Build history of the part. All positions in model axes, mm. Face numbers are marked on the shaded views. A direction names the side the tool comes from. Round coordinates to 2 decimals unless told otherwise and drop trailing zeros. Order: outer loops, then holes, each group sorted by start corner. A loop starts at its lowest first (then second) coordinate and runs counter-clockwise, first axis right, second up. Notation, with made-up numbers: (1, -35.75) - (19, -35.75) arc R20 ccw to (19, -12.75) - close; hole circle Ø8 at (-20.5, 85.25). An arc over 180 degrees is marked (long way). One line per question, with ' | ' between items. Start each with the question number.
from build123d import *

# Parameters (mm, degrees)
SKETCH11_W          = 38.1
SKETCH11_H          = 38.1
SKETCH12_W          = 38.1
SKETCH12_H          = 38.1
BOSS_EXTRUDE5_DEPTH = 12.7
BOSS_EXTRUDE5_TAPER = 20
BOSS_EXTRUDE6_DEPTH = 38.1
SKETCH15_R          = 12.065
CUT_EXTRUDE3_DEPTH  = 25.4
SKETCH16_W          = 23.310601064
SKETCH16_H          = 76.2
CUT_EXTRUDE4_DEPTH  = 59.830675793
SKETCH17_R          = 7.62
BOSS_EXTRUDE7_DEPTH = 6.35
SKETCH18_R          = 5.08
BOSS_EXTRUDE8_DEPTH = 3.81
SKETCH19_R          = 3.1115
BOSS_EXTRUDE9_DEPTH = 7.62
FILLET2_R           = 5.08
SKETCH21_R          = 1.35
CUT_EXTRUDE5_DEPTH  = 63.348983198


with BuildPart() as part:
    # Sweep1: sweep along a path in Sketch10
    with BuildLine(Plane(origin=(0, 0, 0), x_dir=(0, 0, -1), z_dir=(1, 0, 0))) as sweep1_path:
        Line((0, 96.393), (0, -5.207))
        Line((0, -5.207), (-25.324322261, -30.531322261))
    # Sketch11 → Sweep1 (sweep)
    with BuildSketch(Plane(origin=(0, 96.393, 0), x_dir=(1, 0, 0), z_dir=(0, 1, 0))):
        Rectangle(SKETCH11_W, SKETCH11_H)
    sweep(path=sweep1_path.line, transition=Transition.RIGHT)

    # Sketch12 → Boss-Extrude5 (add)
    with BuildSketch(Plane(origin=(0, -27.927822261, 27.927822261), x_dir=(1, 0, 0), z_dir=(0, -0.7071067811865461, 0.7071067811865489))):
        with Locations((0, -3.68190501)):
            Rectangle(SKETCH12_W, SKETCH12_H)
    extrude(amount=BOSS_EXTRUDE5_DEPTH, taper=BOSS_EXTRUDE5_TAPER)

    # Sketch13 → Boss-Extrude6 (add)
    with BuildSketch(Plane(origin=(0, 0, -19.05), x_dir=(-1, 0, 0), z_dir=(0, 0, -1))):
        with BuildLine():
            Line((-19.05, 96.393), (19.05, 96.393))
            ThreePointArc((19.05, 96.393), (0, 115.443), (-19.05, 96.393))
        make_face()
    extrude(amount=-BOSS_EXTRUDE6_DEPTH)

    # Sketch15 → Cut-Extrude3 (cut)
    with BuildSketch(Plane(origin=(0, -36.908078382, 36.908078382), x_dir=(1, 0, 0), z_dir=(0, -0.7071067811865461, 0.7071067811865489))):
        with Locations(Location((0, -3.68190501, 0), (0, 0, 270))):
            Circle(SKETCH15_R)
    extrude(amount=-CUT_EXTRUDE3_DEPTH, mode=Mode.SUBTRACT)

    # Sketch16 → Cut-Extrude4 (cut)
    with BuildSketch(Plane(origin=(19.05, 0, 0), x_dir=(0, 0, -1), z_dir=(1, 0, 0))):
        with Locations((0, 45.72)):
            Rectangle(SKETCH16_W, SKETCH16_H)
    extrude(amount=-CUT_EXTRUDE4_DEPTH, mode=Mode.SUBTRACT)

    # Sketch17 → Boss-Extrude7 (add)
    with BuildSketch(Plane.XY.offset(19.05)):
        with Locations(Location((0, 96.393, 0), (0, 0, 90))):
            Circle(SKETCH17_R)
    extrude(amount=BOSS_EXTRUDE7_DEPTH)

    # Sketch18 → Boss-Extrude8 (add)
    with BuildSketch(Plane.XY.offset(25.4)):
        with Locations(Location((0, 96.393, 0), (0, 0, 180))):
            Circle(SKETCH18_R)
    extrude(amount=BOSS_EXTRUDE8_DEPTH)

    # Sketch19 → Boss-Extrude9 (add)
    with BuildSketch(Plane.XY.offset(29.21)):
        with Locations(Location((0, 96.393, 0), (0, 0, 180))):
            Circle(SKETCH19_R)
    extrude(amount=BOSS_EXTRUDE9_DEPTH)

    # Fillet2
    # the kernel refuses this fillet: 5.08 mm, written as the material it takes off along each edge
    with BuildSketch(Plane(origin=(19.05, 96.393, 19.05), x_dir=(-1, 0, 0), z_dir=(0, -1, 0))) as fillet2_piece_1_section:
        with BuildLine():
            CenterArc((FILLET2_R, FILLET2_R), FILLET2_R, 180, 90)
            Line((0, FILLET2_R), (0, 0))
            Line((0, 0), (FILLET2_R, 0))
        make_face()
    fillet2_piece_1 = extrude(amount=106.409231637, mode=Mode.PRIVATE)
    fillet2_piece_1 = split(fillet2_piece_1, bisect_by=Plane(origin=(17.892257619, 26.96392305, -5.230154687), z_dir=(0, 0.7071067811865489, 0.7071067811865462)), keep=Keep.TOP, mode=Mode.PRIVATE)
    add(fillet2_piece_1, mode=Mode.SUBTRACT)
    with BuildSketch(Plane(origin=(19.05, 96.393, -19.05), x_dir=(0, 0, 1), z_dir=(0, -1, 0))) as fillet2_piece_2:
        with BuildLine():
            CenterArc((FILLET2_R, FILLET2_R), FILLET2_R, 180, 90)
            Line((0, FILLET2_R), (0, 0))
            Line((0, 0), (FILLET2_R, 0))
        make_face()
    extrude(amount=122.190768363, mode=Mode.SUBTRACT)
    with BuildSketch(Plane(origin=(19.05, 11.664024484, 10.069743879), x_dir=(-1, 0, 0), z_dir=(0, -0.7071067811865462, 0.7071067811865489))) as fillet2_piece_3_section:
        with BuildLine():
            CenterArc((FILLET2_R, FILLET2_R), FILLET2_R, 180, 90)
            Line((0, FILLET2_R), (0, 0))
            Line((0, 0), (FILLET2_R, 0))
        make_face()
    fillet2_piece_3 = extrude(amount=53.323231637, mode=Mode.PRIVATE)
    fillet2_piece_3 = split(fillet2_piece_3, bisect_by=Plane(origin=(17.881962417, -12.866336341, 19.05), z_dir=(0, 0, 1)), keep=Keep.TOP, mode=Mode.PRIVATE)
    add(fillet2_piece_3, mode=Mode.SUBTRACT)
    with BuildSketch(Plane(origin=(19.05, -4.117512242, -28.030256121), x_dir=(0, 0.7071067811865489, 0.7071067811865462), z_dir=(0, -0.7071067811865462, 0.7071067811865489))) as fillet2_piece_4:
        with BuildLine():
            CenterArc((FILLET2_R, FILLET2_R), FILLET2_R, 180, 90)
            Line((0, FILLET2_R), (0, 0))
            Line((0, 0), (FILLET2_R, 0))
        make_face()
    extrude(amount=69.104768363, mode=Mode.SUBTRACT)
    with BuildSketch(Plane(origin=(-19.05, -4.117512242, -28.030256121), x_dir=(0, 0.7071067811865488, 0.7071067811865461), z_dir=(0, -0.7071067811865462, 0.7071067811865489))) as fillet2_piece_5:
        with BuildLine():
            CenterArc((FILLET2_R, -FILLET2_R), FILLET2_R, 90, 90)
            Line((0, -FILLET2_R), (0, 0))
            Line((0, 0), (FILLET2_R, 0))
        make_face()
    extrude(amount=69.104768363, mode=Mode.SUBTRACT)
    with BuildSketch(Plane(origin=(-19.05, 11.664024484, 10.069743879), x_dir=(0, -0.7071067811865489, -0.7071067811865462), z_dir=(0, -0.7071067811865462, 0.7071067811865489))) as fillet2_piece_6_section:
        with BuildLine():
            CenterArc((FILLET2_R, FILLET2_R), FILLET2_R, 180, 90)
            Line((0, FILLET2_R), (0, 0))
            Line((0, 0), (FILLET2_R, 0))
        make_face()
    fillet2_piece_6 = extrude(amount=53.323231637, mode=Mode.PRIVATE)
    fillet2_piece_6 = split(fillet2_piece_6, bisect_by=Plane(origin=(-17.881962417, -12.866336341, 19.05), z_dir=(0, 0, 1)), keep=Keep.TOP, mode=Mode.PRIVATE)
    add(fillet2_piece_6, mode=Mode.SUBTRACT)
    with BuildSketch(Plane(origin=(19.05, -15.477476632, 40.378167891), x_dir=(0, 0.7071067811865461, -0.7071067811865488), z_dir=(0, -0.7071067811865489, -0.7071067811865462)), Plane(origin=(-19.05, -45.585167891, 10.270476632), x_dir=(0, 0.7071067811865461, -0.7071067811865489), z_dir=(0, 0.7071067811865489, 0.7071067811865462))) as fillet2_piece_7:
        with BuildLine():
            CenterArc((FILLET2_R * 0.176326980708, -FILLET2_R), FILLET2_R, 90, 20)
            Line((-FILLET2_R * 0.165693162617, -FILLET2_R * 0.0603073792141), (0, 0))
            Line((0, 0), (FILLET2_R * 0.176326980708, 0))
        make_face()
    extrude(amount=42.57870531, mode=Mode.SUBTRACT)
    with BuildSketch(Plane(origin=(-19.05, 96.393, -19.05), x_dir=(0, 0, 1), z_dir=(0, -1, 0))) as fillet2_piece_8:
        with BuildLine():
            CenterArc((FILLET2_R, -FILLET2_R), FILLET2_R, 90, 90)
            Line((0, -FILLET2_R), (0, 0))
            Line((0, 0), (FILLET2_R, 0))
        make_face()
    extrude(amount=122.190768363, mode=Mode.SUBTRACT)
    with BuildSketch(Plane(origin=(-19.05, 96.393, 19.05), x_dir=(1, 0, 0), z_dir=(0, -1, 0))) as fillet2_piece_9_section:
        with BuildLine():
            CenterArc((FILLET2_R, -FILLET2_R), FILLET2_R, 90, 90)
            Line((0, -FILLET2_R), (0, 0))
            Line((0, 0), (FILLET2_R, 0))
        make_face()
    fillet2_piece_9 = extrude(amount=106.409231637, mode=Mode.PRIVATE)
    fillet2_piece_9 = split(fillet2_piece_9, bisect_by=Plane(origin=(-17.892257619, 26.96392305, -5.230154687), z_dir=(0, 0.7071067811865489, 0.7071067811865462)), keep=Keep.TOP, mode=Mode.PRIVATE)
    add(fillet2_piece_9, mode=Mode.SUBTRACT)
    with BuildSketch(Plane(origin=(0, 96.393, -19.05), x_dir=(-1, 0, 0), z_dir=(0, -1, 0))) as fillet2_piece_10:
        with BuildLine():
            CenterArc((19.05 - FILLET2_R, -FILLET2_R), FILLET2_R, 0, 90)
            Line((19.05 - FILLET2_R, 0), (19.05, 0))
            Line((19.05, 0), (19.05, -FILLET2_R))
        make_face()
    revolve(axis=Axis((0, 96.393, -19.05), (0, 0, -1)), revolution_arc=180, mode=Mode.SUBTRACT)
    with BuildSketch(Plane(origin=(0, 96.393, 19.05), x_dir=(-1, 0, 0), z_dir=(0, -1, 0))) as fillet2_piece_11:
        with BuildLine():
            CenterArc((19.05 - FILLET2_R, FILLET2_R), FILLET2_R, 270, 90)
            Line((19.05, FILLET2_R), (19.05, 0))
            Line((19.05, 0), (19.05 - FILLET2_R, 0))
        make_face()
    revolve(axis=Axis((0, 96.393, 19.05), (0, 0, -1)), revolution_arc=180, mode=Mode.SUBTRACT)
    with BuildSketch(Plane(origin=(19.05, 96.393, 19.05), x_dir=(-1, 0, 0), z_dir=(0, -1, 0))) as fillet2_piece_12a_section:
        with BuildLine():
            CenterArc((FILLET2_R, FILLET2_R), FILLET2_R, 180, 90)
            Line((0, FILLET2_R), (0, 0))
            Line((0, 0), (FILLET2_R, 0))
        make_face()
    fillet2_piece_12a = extrude(amount=106.409231637, mode=Mode.PRIVATE)
    fillet2_piece_12a = split(fillet2_piece_12a, bisect_by=Plane(origin=(17.951071981, 0.436282509, 21.297485854), z_dir=(0, -0.7071067811865489, -0.7071067811865462)), keep=Keep.TOP, mode=Mode.PRIVATE)
    with BuildSketch(Plane(origin=(19.05, 11.664024484, 10.069743879), x_dir=(-1, 0, 0), z_dir=(0, -0.7071067811865462, 0.7071067811865489))) as fillet2_piece_12b_section:
        with BuildLine():
            CenterArc((FILLET2_R, FILLET2_R), FILLET2_R, 180, 90)
            Line((0, FILLET2_R), (0, 0))
            Line((0, 0), (FILLET2_R, 0))
        make_face()
    fillet2_piece_12b = extrude(amount=53.323231637, mode=Mode.PRIVATE)
    fillet2_piece_12b = split(fillet2_piece_12b, bisect_by=Plane(origin=(17.951071981, 5.862193339, 19.05), z_dir=(0, 0, -1)), keep=Keep.TOP, mode=Mode.PRIVATE)
    fillet2_piece_12 = fillet2_piece_12a & fillet2_piece_12b
    add(fillet2_piece_12, mode=Mode.SUBTRACT)
    with BuildSketch(Plane(origin=(-19.05, 96.393, 19.05), x_dir=(1, 0, 0), z_dir=(0, -1, 0))) as fillet2_piece_13a_section:
        with BuildLine():
            CenterArc((FILLET2_R, -FILLET2_R), FILLET2_R, 90, 90)
            Line((0, -FILLET2_R), (0, 0))
            Line((0, 0), (FILLET2_R, 0))
        make_face()
    fillet2_piece_13a = extrude(amount=106.409231637, mode=Mode.PRIVATE)
    fillet2_piece_13a = split(fillet2_piece_13a, bisect_by=Plane(origin=(-17.951071981, 0.436282509, 21.297485854), z_dir=(0, -0.7071067811865489, -0.7071067811865462)), keep=Keep.TOP, mode=Mode.PRIVATE)
    with BuildSketch(Plane(origin=(-19.05, 11.664024484, 10.069743879), x_dir=(0, -0.7071067811865489, -0.7071067811865462), z_dir=(0, -0.7071067811865462, 0.7071067811865489))) as fillet2_piece_13b_section:
        with BuildLine():
            CenterArc((FILLET2_R, FILLET2_R), FILLET2_R, 180, 90)
            Line((0, FILLET2_R), (0, 0))
            Line((0, 0), (FILLET2_R, 0))
        make_face()
    fillet2_piece_13b = extrude(amount=53.323231637, mode=Mode.PRIVATE)
    fillet2_piece_13b = split(fillet2_piece_13b, bisect_by=Plane(origin=(-17.951071981, 5.862193339, 19.05), z_dir=(0, 0, -1)), keep=Keep.TOP, mode=Mode.PRIVATE)
    fillet2_piece_13 = fillet2_piece_13a & fillet2_piece_13b
    add(fillet2_piece_13, mode=Mode.SUBTRACT)

    # Sketch21 → Cut-Extrude5 (cut)
    with BuildSketch(Plane(origin=(0, -16.073884182, -16.073884182), x_dir=(1, 0, 0), z_dir=(0, -0.7071067811865486, -0.7071067811865465))):
        with Locations(Location((0, 33.23557837, 0), (0, 0, 270))):
            Circle(SKETCH21_R)
    extrude(amount=-CUT_EXTRUDE5_DEPTH, mode=Mode.SUBTRACT)


solid = part.part
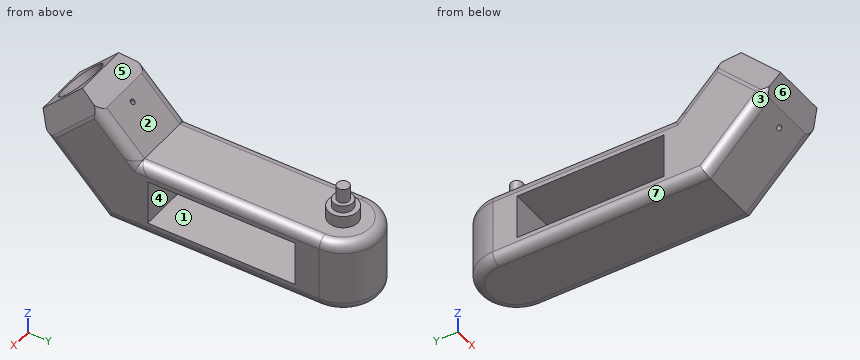
Item 1: Slice it at B-B (z = 9.5). Count the separate pieces of the cut face and the enclosed holes in it, plus the area to 3 significant figures.
Item 2: 3-axis set-ups, long thin cutter, end or side, ignore diameter. For the marked faces 1, 2 and 3: which of +Z, -Z, +X, -X, +Y, -Y reach the whole face in a straight line?
Item 3: Pull direction Y, two halves, no side cores. Call the marked faces 4, 5, 6 and 7: released by +Y, released by -Y, zero draft, split by the parting line, or undercut.
Item 4: Slice it at A-A (y = 64.5). Write the cut outline in (x, z).
Item 5: Pin check, flat tips, straight feed: pin 1 (4 mm diameter, centred on x = 3, y = -22, fed in from +Z); pin 2 (6 mm diameter, centred on x = 3.5, y = 92, fed in from +Z); pin 3 (7 mm diameter, centred on x = 9, z = 2, fed in from -Y). Stop position of each tip, or through.
Item 6: Wall check: line 1 along Z through (x, y) = (-7.5, 28); line 2 along Y through (x, z) = (1, 20). Give the ranges that are in metal, low to high. Write a range as [from, to].
A:
1) separate pieces: 2 | enclosed holes: 2 | area: 2,870 mm^2
2) face 1: +X, -X | face 2: +Z, +X, -X | face 3: -Z, -X, -Y
3) face 4: undercut | face 5: released by +Y | face 6: released by -Y | face 7: zero draft
4) outline: (-19.05, -13.97) arc R5.08 ccw to (-13.97, -19.05) - (13.97, -19.05) arc R5.08 ccw to (19.05, -13.97) - (19.05, -11.66) - (-19.05, -11.66) - close; (-19.05, 11.66) - (19.05, 11.66) - (19.05, 13.97) arc R5.08 ccw to (13.97, 19.05) - (-13.97, 19.05) arc R5.08 ccw to (-19.05, 13.97) - close
5) pin 1: z = 42.03 | pin 2: z = 36.83 | pin 3: y = -37.65
6) line 1: [-19.05, -11.66], [11.66, 19.05] | line 2: [-47.8, -42.21], [-17.9, 1.73], [88.84, 103.95]
